Design review of the part built by this model. Coordinates are the model's own, in mm. A direction names the side the tool comes from. Give positions to 0.01 mm unless a question says otherwise; leave off trailing zeros. Order: outer loops, then holes, each group sorted by start corner. A loop starts at its lowest first (then second) coordinate and runs counter-clockwise, first axis right, second up. Notation, with made-up numbers: (-38, -2.5) -> (1, -2.5) arc R18 ccw to (1, 8.5) -> close; hole circle Ø1 at (47.25, 44.25). An arc over 180 degrees is marked (long way). Use a Markdown table: item, result. Add a question column.
```python
from build123d import *

# Parameters (mm, degrees)
F0_W     = 105.3846
F0_H     = 96.1644
F1_DEPTH = 127
F2_W     = 66.9902929224
F2_H     = 45.6339136045
F3_DEPTH = 155.194


with BuildPart() as f1:
    # F0 (on Front) → F1 (new body)
    with BuildSketch(Plane.XZ):
        Rectangle(F0_W, F0_H)
    extrude(amount=F1_DEPTH)

    # F2 (on face) → F3 (cut, symmetric)
    with BuildSketch(Plane.XZ.offset(127)):
        with Locations((19.1971535388, 25.2652431978)):
            Rectangle(F2_W, F2_H)
    extrude(amount=F3_DEPTH, both=True, mode=Mode.SUBTRACT)


solid = f1.part
```
1) Machinability: for faces 4 (the flat face through (19, -64, 2.448)), 5 (the flat face through (-34, -63, 48.082)), which of the approach directions +Z, -Z, +X, -X, +Y, -Y give a long, thin tool a straight path to every point of the face, cutting with its end or side? Answer none if there is none.
2) Add section C-C (x = 32). Give the boundary of the cut face in (y, z), then the cut area to 3 significant figures.
3) Add section A-A (y = -103.5). Give the boundary of the cut face in (x, z).
4) The part is to be moulded in two halves that separate along Y. For faces 1 (the flat face through (-1, -63, -48.082)), 2 (the flat face through (-12, 0, -10)), 3 (the flat face through (-12, -127, -10)), say which applies: +Y half, -Y half, draft (parallel to the pull), parting line (faces both ways), or undercut.
5) Add section B-B (z = 42.5). Give the boundary of the cut face in (x, y), then the cut area to 3 significant figures.
6) Insertion check: pin 1 (8 mm diameter, centred on x = 39, y = -20, fed in from +Z). The pin has a flat end and moves straight along its axis. Give the tip position at first contact, or say it passes through.
7) For L1, parallel to X at y = -78.5, z = 10.5; L2, parallel to Z at x = 27.5, y = -71, list the stretches that pass through material, from the lowest coordinate up. Write a range as [from, to].
Worked answers:
| question | item | result |
|---|---|---|
| 1 | face 4 | +Z, +X, +Y, -Y |
| 1 | face 5 | +Z, +X, -X, +Y, -Y |
| 2 | outline | (-127, -48.08) -> (0, -48.08) -> (0, 2.45) -> (-127, 2.45) -> close |
| 2 | area | 6,420 mm^2 |
| 3 | outline | (-52.69, -48.08) -> (52.69, -48.08) -> (52.69, 2.45) -> (-14.3, 2.45) -> (-14.3, 48.08) -> (-52.69, 48.08) -> close |
| 4 | face 1 | draft |
| 4 | face 2 | +Y half |
| 4 | face 3 | -Y half |
| 5 | outline | (-52.69, -127) -> (-14.3, -127) -> (-14.3, 0) -> (-52.69, 0) -> close |
| 5 | area | 4,880 mm^2 |
| 6 | pin 1 | z = 2.45 |
| 7 | L1 | [-52.69, -14.3] |
| 7 | L2 | [-48.08, 2.45] |
